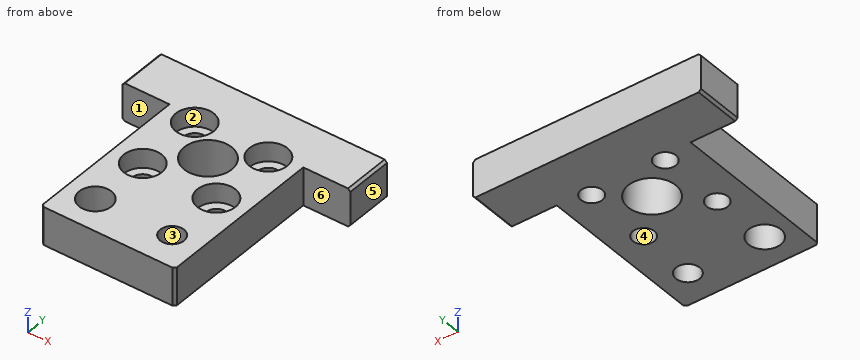
```python
from build123d import *

# Parameters (mm, degrees)
SKETCH1_R             = 5
SKETCH1_R_2           = 2.25
BOSS_EXTRUDE1_DEPTH   = 8
SKETCH2_R             = 4
CUT_EXTRUDE1_DEPTH    = 4
M6_TAPPED_HOLE1_D     = 5
M6_TAPPED_HOLE1_DEPTH = 15
M6_TAPPED_HOLE1_TIP   = 1.502151548
M8_TAPPED_HOLE1_D     = 6.8
M8_TAPPED_HOLE1_DEPTH = 19.75
M8_TAPPED_HOLE1_TIP   = 2.042926105
CHAMFER1_SIZE         = 0.5
CHAMFER2_SIZE         = 0.5


with BuildPart() as part:
    # Sketch1 → Boss-Extrude1 (new body)
    with BuildSketch(Plane.XY):
        Polygon((21.253731343, 11.641791045), (31.164179104, 11.641791045), (31.164179104, 21.641791045), (-16.835820896, 21.641791045), (-16.835820896, 11.641791045), (-6.925373134, 11.641791045), (-6.925373134, -23.358208955), (21.253731343, -23.358208955), align=None)
        with Locations((7.164179104, 3.891791045)):
            Circle(SKETCH1_R, mode=Mode.SUBTRACT)
        with Locations((-0.585820896, -3.858208955)):
            Circle(SKETCH1_R_2, mode=Mode.SUBTRACT)
        with Locations((14.914179104, -3.858208955)):
            Circle(SKETCH1_R_2, mode=Mode.SUBTRACT)
        with Locations((14.914179104, 10.328358209)):
            Circle(SKETCH1_R_2, mode=Mode.SUBTRACT)
        with Locations((-0.585820896, 10.328358209)):
            Circle(SKETCH1_R_2, mode=Mode.SUBTRACT)
    extrude(amount=BOSS_EXTRUDE1_DEPTH)

    # Sketch2 → Cut-Extrude1 (cut)
    with BuildSketch(Plane.XY.offset(8)):
        with Locations((-0.585820896, 10.328358209)):
            Circle(SKETCH2_R)
        with Locations((14.914179104, 10.328358209)):
            Circle(SKETCH2_R)
        with Locations((14.914179104, -3.858208955)):
            Circle(SKETCH2_R)
        with Locations((-0.585820896, -3.858208955)):
            Circle(SKETCH2_R)
    extrude(amount=-CUT_EXTRUDE1_DEPTH, mode=Mode.SUBTRACT)

    # M6 Tapped Hole1
    with Locations(Plane.XY.offset(8)):
        with Locations((15.253731343, -16.358208955)):
            Hole(M6_TAPPED_HOLE1_D / 2, depth=M6_TAPPED_HOLE1_DEPTH)
            with Locations((0, 0, -(M6_TAPPED_HOLE1_DEPTH + M6_TAPPED_HOLE1_TIP / 2))):  # 118° drill point
                Cone(0, M6_TAPPED_HOLE1_D / 2, M6_TAPPED_HOLE1_TIP, mode=Mode.SUBTRACT)

    # M8 Tapped Hole1
    with Locations(Plane.XY.offset(8)):
        with Locations((-0.925373134, -16.358208955)):
            Hole(M8_TAPPED_HOLE1_D / 2, depth=M8_TAPPED_HOLE1_DEPTH)
            with Locations((0, 0, -(M8_TAPPED_HOLE1_DEPTH + M8_TAPPED_HOLE1_TIP / 2))):  # 118° drill point
                Cone(0, M8_TAPPED_HOLE1_D / 2, M8_TAPPED_HOLE1_TIP, mode=Mode.SUBTRACT)

    # Chamfer1
    chamfer1_edges = [part.edges().sort_by_distance(p)[0] for p in [
        (-16.835820896, 16.641791045, 0),
        (31.164179104, 16.641791045, 8),
        (-16.835820896, 16.641791045, 8),
        (31.164179104, 16.641791045, 0),
    ]]
    chamfer(chamfer1_edges, length=CHAMFER1_SIZE)

    # Chamfer2
    chamfer2_edges = [part.edges().sort_by_distance(p)[0] for p in [
        (21.253731343, -23.358208955, 4),
        (-6.925373134, -23.358208955, 4),
    ]]
    chamfer(chamfer2_edges, length=CHAMFER2_SIZE)


solid = part.part
```
Model file for the job. Use its own axes, mm. Face numbers are marked on the shaded views. A direction names the side the tool comes from. Coordinates: 2 decimals unless noted, no trailing zeros. Write each loop counter-clockwise with the first axis right and the second up, starting at its lowest first coordinate (ties: lowest second). Pieces come first, ordered by that corner, then holes. Notation, with made-up numbers: (17.25, 9) - (72.25, 9) arc R36 cw to (72.25, 46) - close; hole circle Ø8 at (87.5, -28). An arc over 180 degrees is marked (long way). One line per item, written item: value. Start each with the question number.
1. Probe line 1 (X direction, y = 10.5, z = 1); line 2 (Y direction, x = 12.5, z = 7.75); line 3 (Y direction, x = 13, z = 6). List the from-to ranges inside material, lowest first. Write a range as from..to.
2. Mould opens along X. For the marked faces 4, 5 and 6 say: released by +X, released by -X, zero draft, split by the parting line, or undercut.
3. Flat gauge pins, fed straight in: pin 1 (6.5 mm diameter, centred on x = -0.59, y = 10.33, fed in from +Z); pin 2 (3 mm diameter, centred on x = 15.25, y = -16.36, fed in from +Z); pin 3 (1.5 mm diameter, centred on y = -9.5, z = 5, fed in from -X); pin 4 (1.5 mm diameter, centred on x = 22, y = 11.5, fed in from +Z). Where does each tip first touch, or does it go through?
4. Tool access for the marked faces 1, 2 and 3: list every direction of +Z, -Z, +X, -X, +Y, -Y with a clear straight run to the whole face (end or side of a thin tool).
5. Slice it at C-C (x = 8). Write the cut outline in (y, z), plus the area to 3 significant figures.
6. Slice it at D-D (x = 15.5). Write the cut outline in (y, z), plus the area to 3 significant figures.
7. Slice it at B-B (z = 1.75). Write the cut outline in (x, y).
8. Slice it at A-A (y = 3). Write the cut outline in (x, z), plus the area to 3 significant figures.
Answers below:
1. line 1: x = -6.93..-2.83, 1.66..12.67, 17.16..21.25
1. line 2: y = -23.36..-7.05, -0.67..7.14, 13.52..21.64
1. line 3: y = -23.36..-17.44, -15.28..-7.37, -0.35..6.82, 13.84..21.64
2. face 4: undercut
2. face 5: released by +X
2. face 6: zero draft
3. pin 1: stops at z = 4
3. pin 2: passes through
3. pin 3: stops at x = -6.93
3. pin 4: stops at z = 8
4. face 1: +Z, -Z, -X, -Y
4. face 2: +Z
4. face 3: +Z, -Z
5. outline: (-23.36, 0) - (-1.04, 0) - (-1.04, 8) - (-23.36, 8) - close; (8.82, 0) - (21.64, 0) - (21.64, 8) - (8.82, 8) - close
5. area: 281 mm^2
6. outline: (-23.36, 0) - (-18.85, 0) - (-18.85, 8) - (-23.36, 8) - close; (-13.87, 0) - (-6.03, 0) - (-6.03, 4) - (-7.82, 4) - (-7.82, 8) - (-13.87, 8) - close; (-1.69, 0) - (8.16, 0) - (8.16, 4) - (6.37, 4) - (6.37, 8) - (0.1, 8) - (0.1, 4) - (-1.69, 4) - close; (12.5, 0) - (21.64, 0) - (21.64, 8) - (14.29, 8) - (14.29, 4) - (12.5, 4) - close
6. area: 222 mm^2
7. outline: (-16.84, 11.64) - (-6.93, 11.64) - (-6.93, -22.86) - (-6.43, -23.36) - (20.75, -23.36) - (21.25, -22.86) - (21.25, 11.64) - (31.16, 11.64) - (31.16, 21.64) - (-16.84, 21.64) - close; hole circle Ø6.8 at (-0.93, -16.36); hole circle Ø4.5 at (-0.59, -3.86); hole circle Ø4.5 at (-0.59, 10.33); hole circle Ø10 at (7.16, 3.89); hole circle Ø4.5 at (14.91, -3.86); hole circle Ø4.5 at (14.91, 10.33); hole circle Ø5 at (15.25, -16.36)
8. outline: (-6.93, 0) - (2.24, 0) - (2.24, 8) - (-6.93, 8) - close; (12.08, 0) - (21.25, 0) - (21.25, 8) - (12.08, 8) - close
8. area: 147 mm^2
